For this review, use the dimensioned drawing (mm, ordinates from the lowest corner) and the shaded views. Round coordinates to 2 decimals unless told otherwise and drop trailing zeros. Write each loop counter-clockwise with the first axis right and the second up, starting at its lowest first coordinate (ties: lowest second). Pieces come first, ordered by that corner, then holes. Notation, with made-up numbers: M -10,-3.75 L 17,-3.75 A31 cw 17,33.25 Z; hole C 2,-35 d5. An arc over 180 degrees is marked long. One line per question, with ' | ' between items. Start each with the question number.
Item 1: Add section D-D, the plane x = 96. State the section outline as (y, z) points, and give its area (3 significant figures).
Item 2: Add section A-A, the plane y = 50. State the section outline as (x, z) points.
Item 3: Add section C-C, the plane z = 1.7. Give the number of separate pieces and of enclosed holes in the cut face, and give its area (3 significant figures).
Item 4: For L1, parallel to X at y = 37.5, z = 1.6 (1 decimal); L2, parallel to X at y = 23, z = 1.65 (1 decimal); L3, parallel to Y at x = 44, z = 0.2, list the stretches that pass through material, from the lowest coordinate up.
Item 5: Add section B-B, the plane x = 50. State the section outline as (y, z) points, and give its area (3 significant figures).
Item 6: Insertion check: pin 1 Ø4 at (x, y) = (35, 65.5) entering from -Z; pin 2 Ø1.5 at (x, z) = (13.5, 2) entering from +Y (1 decimal). Each pin has a flat end and moves straight along its axis. Give the tip position at first contact, or say it passes through.
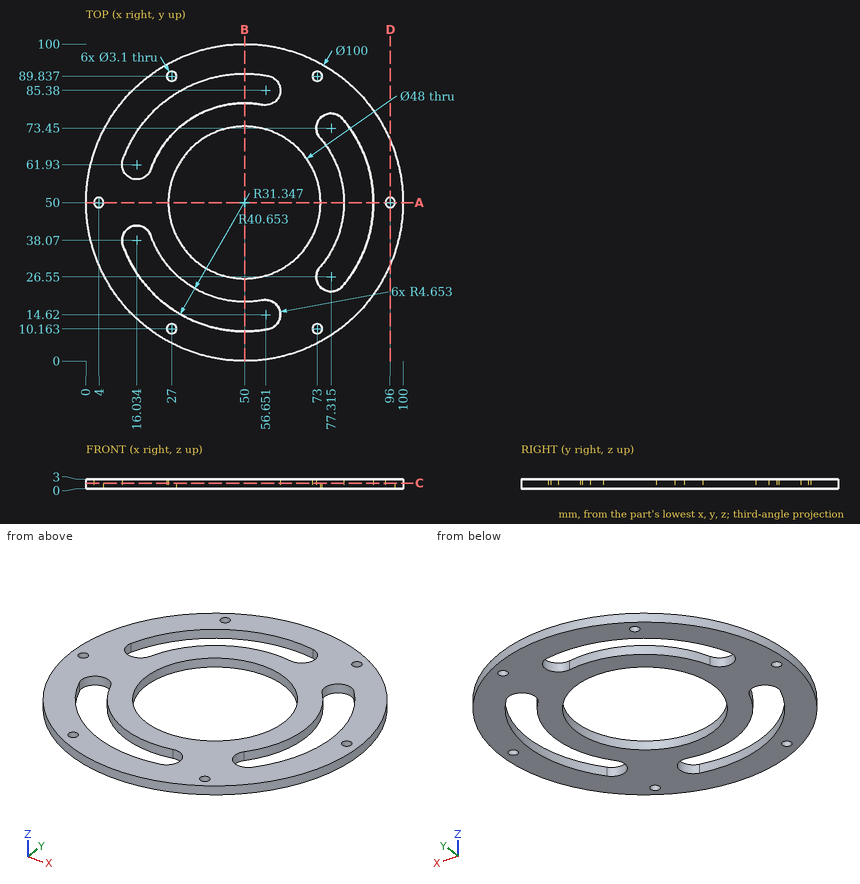
Computed values:
1) outline: M 30.4,0 L 48.45,0 L 48.45,3 L 30.4,3 Z; M 51.55,0 L 69.6,0 L 69.6,3 L 51.55,3 Z | area: 108 mm^2
2) outline: M 0,0 L 2.45,0 L 2.45,3 L 0,3 Z; M 5.55,0 L 26,0 L 26,3 L 5.55,3 Z; M 74,0 L 81.35,0 L 81.35,3 L 74,3 Z; M 90.65,0 L 94.45,0 L 94.45,3 L 90.65,3 Z; M 97.55,0 L 100,0 L 100,3 L 97.55,3 Z
3) separate pieces: 1 | enclosed holes: 10 | area: 4,370 mm^2
4) L1: x = 1.6 to 11.4, 21.3 to 29.5, 70.5 to 78.7, 88.7 to 98.4 | L2: x = 7.9 to 19.6, 34.1 to 74.3, 80.3 to 92.1 | L3: y = 0.36 to 9.79, 19.23 to 26.76, 73.24 to 80.77, 90.21 to 99.64
5) outline: M 0,0 L 9.35,0 L 9.35,3 L 0,3 Z; M 18.65,0 L 26,0 L 26,3 L 18.65,3 Z; M 74,0 L 81.35,0 L 81.35,3 L 74,3 Z; M 90.65,0 L 100,0 L 100,3 L 90.65,3 Z | area: 100 mm^2
6) pin 1: passes through | pin 2: stops at y = 85
